Part model, mm, in its own coordinate system. A direction names the side the tool comes from. Give positions to 0.01 mm unless a question says otherwise; leave off trailing zeros. Write each loop counter-clockwise with the first axis right and the second up, starting at its lowest first coordinate (ties: lowest second). Pieces come first, ordered by that corner, then holes. Notation, with made-up numbers: M 62.5,49 L 78.5,49 A34 ccw 78.5,88 Z; hole C -35,-20.5 d10. An arc over 180 degrees is marked long. Answer as CSV lines item,"result". Start each with the question number.
1) Slice it at C-C, the plane x = 0. Give the cut face in (y, z).
2) Mould opens along Y. For faces 3 (the cylindrical face through (-20.961, -15.686, -12.748)), 4 (the flat face through (14.976, -1.489, -23.986)), 5 (the flat face through (-2, 11.213, -12)), 6 (the cylindrical face through (9.5, 5, -0.3)) say: pulls with the +Y half, pulls with the -Y half, needs draft (parallel to the pull), parting line crosses it, or undercut.
3) Tool access for faces 1 (the flat face through (-3, -16.287, -12)), 2 (the cylindrical face through (-13.832, -1.098, -0.285)): list every direction of +Z, -Z, +X, -X, +Y, -Y with a clear straight run to the whole face (end or side of a thin tool).
4) Pin check, flat tips, straight feed: pin 1 Ø7.5 at (x, y) = (9.5, -2.5) entering from +Z; pin 2 Ø3.5 at (x, y) = (-17, 3) entering from +Z; pin 3 Ø2.5 at (x, y) = (-12, 0) entering from +Z. Stop position of each tip, or through.
5) Wall check: line 1 along X through (y, z) = (4.75, -8); line 2 along X through (y, z) = (-7, -4.25); line 3 along Y through (x, z) = (1, -4.5). Give the ranges that are in metal, low to high. Write a range as from..to.
6) Slice it at A-A, the plane y = 8.5. Give the cut face in (x, z).
7) Slice it at B-B, the plane z = -12.25. Give the cut face in (x, y), plus the area to 3 significant figures.
```python
from build123d import *

# Parameters (mm, degrees)
F0_W     = 37
F0_H     = 30
F0_W_2   = 3
F0_H_2   = 25
F0_W_3   = 9
F0_W_4   = 7
F0_H_3   = 12
F1_DEPTH = 25
F2_DEPTH = 22.5
F3_SIZE2 = 2
F3_SIZE  = 1
F4_R     = 2
F5_R     = 1


with BuildPart() as f1:
    # F0 (on Top) → F1 (new body)
    with BuildSketch(Plane.XY):
        with Locations((-3.031099186, -1.2872133628)):
            Rectangle(F0_W, F0_H)
        with Locations((-17.531099186, -1.2872133628)):
            Rectangle(F0_W_2, F0_H_2, mode=Mode.SUBTRACT)
        with Locations((-12.031099186, -1.2872133628)):
            Rectangle(F0_W_2, F0_H_2, mode=Mode.SUBTRACT)
        with Locations((-2.031099186, -1.2872133628)):
            Rectangle(F0_W_3, F0_H_2, mode=Mode.SUBTRACT)
        with Locations((9.468900814, -1.2872133628)):
            Rectangle(F0_W_4, F0_H_3, mode=Mode.SUBTRACT)
        with Locations((-17.531099186, -1.2872133628)):
            Rectangle(F0_W_2, F0_H_2)
        with Locations((-12.031099186, -1.2872133628)):
            Rectangle(F0_W_2, F0_H_2)
        with Locations((-2.031099186, -1.2872133628)):
            Rectangle(F0_W_3, F0_H_2)
        with Locations((9.468900814, -1.2872133628)):
            Rectangle(F0_W_4, F0_H_3)
    extrude(amount=-F1_DEPTH)

    # F0 (on Top) → F2 (cut)
    with BuildSketch(Plane.XY):
        with Locations((-17.531099186, -1.2872133628)):
            Rectangle(F0_W_2, F0_H_2)
        with Locations((-12.031099186, -1.2872133628)):
            Rectangle(F0_W_2, F0_H_2)
        with Locations((-2.031099186, -1.2872133628)):
            Rectangle(F0_W_3, F0_H_2)
        with Locations((9.468900814, -1.2872133628)):
            Rectangle(F0_W_4, F0_H_3)
    extrude(amount=-F2_DEPTH, mode=Mode.SUBTRACT)

    # F3
    f3_edges = [f1.edges().sort_by_distance(p)[0] for p in [
        (-3.031099, -16.287213, -25),
        (15.468901, -1.287213, -25),
        (-3.031099, 13.712787, -25),
        (-21.531099, -1.287213, -25),
    ]]
    f3_side = f1.faces().sort_by_distance((-3.031099, -1.287213, -25))[0]
    chamfer(f3_edges, length=F3_SIZE, length2=F3_SIZE2, reference=f3_side)

    # F4
    f4_edges = [f1.edges().sort_by_distance(p)[0] for p in [
        (-21.531099, -16.287213, -11.5),
        (-21.531099, 13.712787, -11.5),
        (15.468901, 13.712787, -11.5),
        (15.468901, -16.287213, -11.5),
    ]]
    fillet(f4_edges, radius=F4_R)

    # F5
    f5_edges = [f1.edges().sort_by_distance(p)[0] for p in [
        (12.968901, -1.287213, 0),
        (9.468901, -7.287213, 0),
        (5.968901, -1.287213, 0),
        (9.468901, 4.712787, 0),
        (2.468901, -1.287213, 0),
        (-2.031099, -13.787213, 0),
        (-6.531099, -1.287213, 0),
        (-2.031099, 11.212787, 0),
        (-10.531099, -1.287213, 0),
        (-12.031099, -13.787213, 0),
        (-13.531099, -1.287213, 0),
        (-12.031099, 11.212787, 0),
        (-16.031099, -1.287213, 0),
        (-17.531099, 11.212787, 0),
        (-19.031099, -1.287213, 0),
        (-17.531099, -13.787213, 0),
        (-3.031099, 13.712787, 0),
    ]]
    fillet(f5_edges, radius=F5_R)


solid = f1.part
```
Found:
1,outline,"M -16.29,-23 L -15.29,-25 L 12.71,-25 L 13.71,-23 L 13.71,-1 A1 ccw 12.71,0 L 12.21,0 A1 ccw 11.21,-1 L 11.21,-22.5 L -13.79,-22.5 L -13.79,-1 A1 ccw -14.79,0 L -15.29,0 A1 ccw -16.29,-1 Z"
2,face 3,"pulls with the -Y half"
2,face 4,"needs draft"
2,face 5,"undercut"
2,face 6,"undercut"
3,face 1,"+Z, -Z, +X, -X, -Y"
3,face 2,"+Z"
4,pin 1,"z = -0.3"
4,pin 2,"z = -0.02"
4,pin 3,"z = -22.5"
5,line 1,"-21.53..-19.03, -16.03..-13.53, -10.53..-6.53, 2.47..15.47"
5,line 2,"-21.53..-19.03, -16.03..-13.53, -10.53..-6.53, 2.47..5.97, 12.97..15.47"
5,line 3,"-16.29..-13.79, 11.21..13.71"
6,outline,"M -21.53,-23 L -20.53,-25 L 14.47,-25 L 15.47,-23 L 15.47,-1 A1 ccw 14.47,0 L 3.47,0 A1 ccw 2.47,-1 L 2.47,-22.5 L -6.53,-22.5 L -6.53,-1 A1 ccw -7.53,0 L -9.53,0 A1 ccw -10.53,-1 L -10.53,-22.5 L -13.53,-22.5 L -13.53,-1 A1 ccw -14.53,0 L -15.03,0 A1 ccw -16.03,-1 L -16.03,-22.5 L -19.03,-22.5 L -19.03,-1 A1 ccw -20.03,0 L -20.53,0 A1 ccw -21.53,-1 Z"
7,outline,"M -21.53,-14.29 A2 ccw -19.53,-16.29 L 13.47,-16.29 A2 ccw 15.47,-14.29 L 15.47,11.71 A2 ccw 13.47,13.71 L -19.53,13.71 A2 ccw -21.53,11.71 Z; hole M -19.03,-13.79 L -16.03,-13.79 L -16.03,11.21 L -19.03,11.21 Z; hole M -13.53,-13.79 L -10.53,-13.79 L -10.53,11.21 L -13.53,11.21 Z; hole M -6.53,-13.79 L 2.47,-13.79 L 2.47,11.21 L -6.53,11.21 Z; hole M 5.97,-7.29 L 12.97,-7.29 L 12.97,4.71 L 5.97,4.71 Z"
7,area,"648 mm²"
